Build history of the part. All positions in model axes, mm. Round coordinates to 2 decimals unless told otherwise and drop trailing zeros. Loops run counter-clockwise (first coordinate to the right, second up) from the corner with the lowest first, then second, coordinate; pieces in that order, holes last.
from build123d import *

# Parameters (mm, degrees)
SKETCH4_R           = 14.58
SKETCH4_R_2         = 9.58
BOSS_EXTRUDE1_DEPTH = 15
SKETCH5_R           = 14.58
SKETCH5_R_2         = 14.38
CUT_EXTRUDE1_DEPTH  = 31


with BuildPart() as part:
    # Sketch2 → Revolve1 (revolve)
    with BuildSketch(Plane.XY):
        with BuildLine():
            Line((9.58, 0), (14.58, 0))
            Line((14.58, 0), (14.58, -10.882649731))
            ThreePointArc((14.58, -10.882649731), (14.446025404, -11.382649731), (14.08, -11.748675135))
            Line((14.08, -11.748675135), (11.08, -13.480725942))
            ThreePointArc((11.08, -13.480725942), (10.08, -13.480725942), (9.58, -12.614700538))
            Line((9.58, -12.614700538), (9.58, 0))
        make_face()
    revolve(axis=Axis((0, 0, 0), (0, -1, 0)))

    # Sketch4 → Boss-Extrude1 (add)
    with BuildSketch(Plane(origin=(0, 0, 0), x_dir=(1, 0, 0), z_dir=(0, 1, 0))):
        Circle(SKETCH4_R)
        Circle(SKETCH4_R_2, mode=Mode.SUBTRACT)
    extrude(amount=BOSS_EXTRUDE1_DEPTH)

    # Sketch5 → Cut-Extrude1 (cut)
    with BuildSketch(Plane(origin=(0, 15, 0), x_dir=(1, 0, 0), z_dir=(0, 1, 0))):
        Circle(SKETCH5_R)
        Circle(SKETCH5_R_2, mode=Mode.SUBTRACT)
    extrude(amount=-CUT_EXTRUDE1_DEPTH, mode=Mode.SUBTRACT)


solid = part.part
(1) Pull direction X, two halves, no side cores. Call faces 1 (the face through (-2.08, 1, 9.35)), 2 (the face through (3, 15, 9.4)), 3 (the face through (-3.117, 1.944, 14.038)): +X half, -X half, draft (parallel to the pull), parting line (faces both ways), or undercut.
Responses:
face 1: undercut
face 2: draft
face 3: parting line
(2) Probe line 1 (Z direction, x = 0, y = -1); line 2 (Z direction, x = -8, y = -4.75). List the from-to ranges inside material, lowest first.
Responses:
line 1: z = -14.38 to -9.58, 9.58 to 14.38
line 2: z = -11.95 to -5.27, 5.27 to 11.95
(3) Slice it at C-C on y = -0.5. List the corners of the cut face in (x, z), plus the area to 3 significant figures.
Responses:
outline: circle Ø28.76 at (0, 0); hole circle Ø19.16 at (0, 0)
area: 361 mm2
(4) Slice it at A-A on x = 0. List the corners of the cut face in (y, z), plus the area to 3 significant figures.
Responses:
outline: (-13.48, -11.08) - (-11.75, -14.08) arc R1 ccw to (-11.48, -14.38) - (15, -14.38) - (15, -9.58) - (-12.61, -9.58) arc R1 ccw to start; (-13.48, 11.08) arc R1 ccw to (-12.61, 9.58) - (15, 9.58) - (15, 14.38) - (-11.48, 14.38) arc R1 ccw to (-11.75, 14.08) - close
area: 267 mm2
(5) Pin check, flat tips, straight feed: P1, Ø15.5, axis at x = 0, z = 0, coming from the -Y side; P2, Ø1.5, axis at x = -3, y = 11, coming from the +Z side; P3, Ø3, axis at x = -4.5, y = 9, coming from the +Z side; P4, Ø3, axis at x = 9.5, y = -4.5, coming from the +Z side. Stop position of each tip, or through.
Responses:
P1: passes through
P2: stops at z = 14.2
P3: stops at z = 14.06
P4: stops at z = 11.95
(6) Slice it at B-B on z = 0. List the corners of the cut face in (x, y), plus the area to 3 significant figures.
Responses:
outline: (-14.38, -11.48) arc R1 ccw to (-14.08, -11.75) - (-11.08, -13.48) arc R1 ccw to (-9.58, -12.61) - (-9.58, 15) - (-14.38, 15) - close; (9.58, -12.61) arc R1 ccw to (11.08, -13.48) - (14.08, -11.75) arc R1 ccw to (14.38, -11.48) - (14.38, 15) - (9.58, 15) - close
area: 267 mm2
